```python
from build123d import *

# Parameters (mm, degrees)
SKETCH_1_R          = 9
SKETCH_1_R_2        = 8
EXTRUDE_1_DEPTH     = 95
EXTRUDE_2_DEPTH     = 10
EXTRUDE_3_DEPTH     = 12
SKETCH_4_R          = 5
EXTRUDE_4_DEPTH     = 8
SKETCH_5_R          = 2.5
CUT_EXTRUDE_1_DEPTH = 38
SKETCH_6_R          = 2
SKETCH_6_R_2        = 1.980516498
CUT_EXTRUDE_3_DEPTH = 3


with BuildPart() as part:
    # 草图1 → 凸台-拉伸1 (new body)
    with BuildSketch(Plane.XY):
        Circle(SKETCH_1_R)
        Circle(SKETCH_1_R_2, mode=Mode.SUBTRACT)
    extrude(amount=EXTRUDE_1_DEPTH)

    # 草图2 → 凸台-拉伸2 (add)
    with BuildSketch(Plane.XY.offset(95)):
        with BuildLine():
            Line((-5, -9), (5, -9))
            ThreePointArc((5, -9), (7.828427125, -7.828427125), (9, -5))
            Line((9, -5), (9, 5))
            ThreePointArc((9, 5), (7.828427125, 7.828427125), (5, 9))
            Line((5, 9), (-5, 9))
            ThreePointArc((-5, 9), (-7.828427125, 7.828427125), (-9, 5))
            Line((-9, 5), (-9, -5))
            ThreePointArc((-9, -5), (-7.828427125, -7.828427125), (-5, -9))
        make_face()
    extrude(amount=EXTRUDE_2_DEPTH)

    # 草图3 → 凸台-拉伸3 (add)
    with BuildSketch(Plane(origin=(0, 0, 0), x_dir=(-1, 0, 0), z_dir=(0, 0, -1))):
        with BuildLine():
            Line((-5, -9), (5, -9))
            ThreePointArc((5, -9), (7.828427125, -7.828427125), (9, -5))
            Line((9, -5), (9, 5))
            ThreePointArc((9, 5), (7.828427125, 7.828427125), (5, 9))
            Line((5, 9), (-5, 9))
            ThreePointArc((-5, 9), (-7.828427125, 7.828427125), (-9, 5))
            Line((-9, 5), (-9, -5))
            ThreePointArc((-9, -5), (-7.828427125, -7.828427125), (-5, -9))
        make_face()
    extrude(amount=EXTRUDE_3_DEPTH)

    # 草图4 → 凸台-拉伸4 (add)
    with BuildSketch(Plane(origin=(0, 0, -12), x_dir=(-1, 0, 0), z_dir=(0, 0, -1))):
        Circle(SKETCH_4_R)
    extrude(amount=EXTRUDE_4_DEPTH)

    # 草图5 → 切除-拉伸1 (cut)
    with BuildSketch(Plane(origin=(0, 0, -20), x_dir=(-1, 0, 0), z_dir=(0, 0, -1))):
        Circle(SKETCH_5_R)
    extrude(amount=-CUT_EXTRUDE_1_DEPTH, mode=Mode.SUBTRACT)

    # 草图6 → 切除-拉伸3 (cut)
    with BuildSketch(Plane.ZY.offset(9)):
        with Locations((-4, 0)):
            Circle(SKETCH_6_R)
        with Locations((99, 0)):
            Circle(SKETCH_6_R_2)
    extrude(amount=-CUT_EXTRUDE_3_DEPTH, mode=Mode.SUBTRACT)


solid = part.part
```
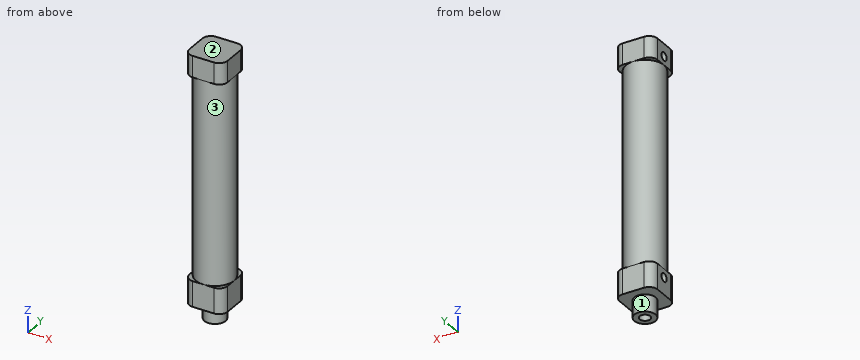
Here's how the part is built. I have some questions about the finished solid (model axes, mm). Face numbers are marked on the shaded views. Round coordinates to 2 decimals unless told otherwise and drop trailing zeros. Loops run counter-clockwise (first coordinate to the right, second up) from the corner with the lowest first, then second, coordinate; pieces in that order, holes last.
1. If I drill on probe 1 along Y at (x, z) = (0, -4.5); probe 2 along Z at (x, y) = (-2, -7.5); probe 3 along Y at (x, z) = (0, 54), over which ranges is the centre line in solid material (lowest first)?
Answers:
probe 1: y = -9 to -2.5, 2.5 to 9
probe 2: z = -12 to 0, 95 to 105
probe 3: y = -9 to -8, 8 to 9
2. Suppose I cut it at B-B, the plane z = 99. Please give me the cut outline in (x, y), and give its area (3 significant figures).
Answers:
outline: (-9, -5) arc R4 ccw to (-5, -9) - (5, -9) arc R4 ccw to (9, -5) - (9, 5) arc R4 ccw to (5, 9) - (-5, 9) arc R4 ccw to (-9, 5) - (-9, 1.98) - (-6, 1.98) - (-6, -1.98) - (-9, -1.98) - close
area: 298 mm2
3. Thinking about a two-plate mould opening in Z: for the marked faces 1, 2 and 3, which applies, released by +Z, released by -Z, zero draft, split by the parting line, or undercut?
Answers:
face 1: zero draft
face 2: released by +Z
face 3: undercut
4. Suppose I cut it at C-C, the plane z = 20. Please give me the cut outline in (x, y).
Answers:
outline: circle Ø18 at (0, 0); hole circle Ø16 at (0, 0)
5. Will these pins go through, and if not, where does the flat tip stop? pin 1 (6 mm diameter, centred on x = -6.5, z = 53, fed in from -Y); pin 2 (10 mm diameter, centred on x = 0.5, z = 66, fed in from -Y); pin 3 (2 mm diameter, centred on x = -3.5, z = 18.5, fed in from +Y); pin 4 (4 mm diameter, centred on x = 5, y = 6.5, fed in from -Z).
Answers:
pin 1: stops at y = -8.29
pin 2: stops at y = -9
pin 3: stops at y = 8.65
pin 4: stops at z = -12
6. Suppose I cut it at A-A, the plane z = -4. Please give me the cut outline in (x, y).
Answers:
outline: (-9, -5) arc R4 ccw to (-5, -9) - (5, -9) arc R4 ccw to (9, -5) - (9, 5) arc R4 ccw to (5, 9) - (-5, 9) arc R4 ccw to (-9, 5) - (-9, 2) - (-6, 2) - (-6, -2) - (-9, -2) - close; hole circle Ø5 at (0, 0)
